Verification items for the finished model (mm, model axes). A direction names the side the tool comes from. Round coordinates to 2 decimals unless told otherwise and drop trailing zeros. Write each loop counter-clockwise with the first axis right and the second up, starting at its lowest first coordinate (ties: lowest second). Pieces come first, ordered by that corner, then holes. Notation, with made-up numbers: M -14,5.5 L -3,5.5 A16 ccw -3,33.5 Z; hole C 34,-9 d9. An arc over 180 degrees is marked long. Write each question's results on one line, items separated by ' | '.
Autodesk Inventor part; units mm, degrees
ref_plane "YZ Plane" through (0, 0, 0) normal (1, 0, 0) x (0, 1, 0)
ref_plane "XZ Plane" through (0, 0, 0) normal (0, 1, 0) x (-1, 0, 0)
ref_plane "XY Plane" through (0, 0, 0) normal (0, 0, 1) x (1, 0, 0)
sketch "Sketch1" plane through (0, 0, 0) normal (1, 0, 0) x (0, 1, 0)
  circle A0 centre (0, 0) radius 22.5
  dimension "d0" = 45
extrude "Extrusion1" add sketch "Sketch1" along normal blind 110
sketch "Sketch2" plane through (110, 0, 0) normal (1, 0, 0) x (0, 0, -1)
  line L0 (2.5, 26.6733) -> (-2.5, 26.6733)
  line L1 (-2.5, 26.6733) -> (-2.5, -26.6733)
  line L2 (-2.5, -26.6733) -> (2.5, -26.6733)
  line L3 (2.5, -26.6733) -> (2.5, 26.6733)
  line L4 (2.5, 26.6733) -> (-2.5, -26.6733) construction
  line L5 (-2.5, 26.6733) -> (2.5, -26.6733) construction
  circle A0 centre (0, 0) radius 2.5
  dimension "d3" = 5
  dimension "d12" = 5
extrude "Extrusion2" cut sketch "Sketch2" against normal blind 5
sketch "Sketch4" plane through (0, 0, 0) normal (-1, 0, 0) x (0, 0, 1)
  line L0 (-2.5, -27.3209) -> (2.5, -27.3209)
  line L1 (2.5, -27.3209) -> (2.5, 27.3209)
  line L2 (2.5, 27.3209) -> (-2.5, 27.3209)
  line L3 (-2.5, 27.3209) -> (-2.5, -27.3209)
  line L4 (-2.5, -27.3209) -> (2.5, 27.3209) construction
  line L5 (2.5, -27.3209) -> (-2.5, 27.3209) construction
  point P0 (0, 0)
  dimension "d9" = 5
extrude "Extrusion4" cut sketch "Sketch4" against normal blind 5
sketch "Sketch5" plane through (105, 0, 0) normal (1, 0, 0) x (0, 0, -1)
  circle A0 centre (0, 0) radius 2.5
  dimension "d13" = 5
extrude "Extrusion5" cut sketch "Sketch5" against normal blind 110
properties part number "Conveyor Belt Shaft" material "Stainless Steel AISI 440C, Welded"
1) Sectioned sample at D-D, the plane y = -4. Record the cut outline in (x, z).
Calculated:
outline: M 0,-22.14 L 110,-22.14 L 110,-2.5 L 105,-2.5 L 105,2.5 L 110,2.5 L 110,22.14 L 0,22.14 L 0,2.5 L 5,2.5 L 5,-2.5 L 0,-2.5 Z
2) Material ranges on line 1 (Y direction, x = 58.5, z = 15.5); line 2 (Z direction, x = 103, y = 9.5); line 3 (X direction, y = -16.5, z = -1.5), recorded low to high. Write a range as [from, to].
Calculated:
line 1: y = [-16.31, 16.31] | line 2: z = [-20.4, 20.4] | line 3: x = [5, 105]
3) Draft check along Z on faces 4 (the flat face through (5, -11, 0)), 5 (the flat face through (110, 0, -10)), 6 (the cylindrical face through (54.23, 10.382, 19.961)). Enter one of: pulls with the +Z half, pulls with the -Z half, needs draft (parallel to the pull), parting line crosses it, or undercut.
Calculated:
face 4: undercut | face 5: needs draft | face 6: parting line crosses it
4) Sectioned sample at B-B, the plane y = 18. Record the cut outline in (x, z).
Calculated:
outline: M 0,-13.5 L 110,-13.5 L 110,-2.5 L 105,-2.5 L 105,2.5 L 110,2.5 L 110,13.5 L 0,13.5 L 0,2.5 L 5,2.5 L 5,-2.5 L 0,-2.5 Z
5) Sectioned sample at C-C, the plane x = 82.5. Record the cut outline in (y, z), and give its area (3 significant figures).
Calculated:
outline: C 0,0 d45; hole C 0,0 d5 | area: 1,570 mm²
6) Access from +Z, -Z, +X, -X, +Y, -Y to the whole of each face (thin tool, end or side, straight path). Record for faces 1 (the flat face through (108, 0, 2.5)), 2 (the flat face through (2, 0, -2.5)), 3 (the flat face through (0, 0, 10)).
Calculated:
face 1: +X, +Y, -Y | face 2: -X, +Y, -Y | face 3: +Z, -Z, -X, +Y, -Y
7) Sectioned sample at A-A, the plane z = 0. Record the cut outline in (x, y).
Calculated:
outline: M 5,-22.5 L 105,-22.5 L 105,-2.5 L 5,-2.5 Z; M 5,2.5 L 105,2.5 L 105,22.5 L 5,22.5 Z
8) Depth check by flat-ended pin: P1, Ø5.5, axis at y = 13, z = 0, coming from the -X side; P2, Ø4, axis at x = 59.5, z = -7, coming from the -Y side; P3, Ø3, axis at x = 86, z = 14, coming from the -Y side; P4, Ø1.5, axis at y = -10, z = -1, coming from the +X side. Enter the tip coordinate at first touch or a pass-through.
Calculated:
P1: stops at x = 0 | P2: stops at y = -21.94 | P3: stops at y = -18.71 | P4: stops at x = 105
